Read the model definition and answer for the solid it produces. Units are mm, in the model's axes. A direction names the side the tool comes from. Round coordinates to 2 decimals unless told otherwise and drop trailing zeros. Loops run counter-clockwise (first coordinate to the right, second up) from the corner with the lowest first, then second, coordinate; pieces in that order, holes last. Notation, with made-up numbers: (2, -23.5) - (31, -23.5) arc R31 ccw to (31, 3.5) - close; hole circle Ø4 at (-21, -29). An arc over 180 degrees is marked (long way). Answer as CSV lines item,"result".
```python
from build123d import *

# Parameters (mm, degrees)
F1_DEPTH = 101.6


with BuildPart() as f1:
    # F0 (on Front) → F1 (new body)
    with BuildSketch(Plane.XZ):
        Polygon((-50.8, -32.374417), (50.8, -32.374417), (50.8, 32.374417), (14.084613, 32.374417), (-50.8, 32.374417), align=None)
        with BuildLine():
            Line((14.084613, 32.374417), (50.8, 32.374417))
            Line((50.8, 32.374417), (50.8, 52.120494))
            Line((50.8, 52.120494), (50.8, 74.345494))
            ThreePointArc((50.8, 74.345494), (24.954765, 64.252521), (14.084613, 38.724417))
            Line((14.084613, 38.724417), (14.084613, 32.374417))
        make_face()
        with BuildLine():
            ThreePointArc((50.8, 74.345494), (-5.45833, 66.573015), (-50.8, 32.374417))
            Line((-50.8, 32.374417), (14.084613, 32.374417))
            Line((14.084613, 32.374417), (14.084613, 38.724417))
            ThreePointArc((14.084613, 38.724417), (24.954765, 64.252521), (50.8, 74.345494))
        make_face()
        with BuildLine():
            Line((50.8, 74.345494), (50.8, 52.120494))
            Line((50.8, 52.120494), (90.314029, 52.120494))
            ThreePointArc((90.314029, 52.120494), (94.804157, 53.980366), (96.664029, 58.470494))
            Line((96.664029, 58.470494), (96.664029, 102.920494))
            Line((96.664029, 102.920494), (57.15, 102.920494))
            ThreePointArc((57.15, 102.920494), (52.659872, 101.060622), (50.8, 96.570494))
            Line((50.8, 96.570494), (50.8, 74.345494))
        make_face()
    extrude(amount=F1_DEPTH)


solid = f1.part
```
1) A cutting plane is placed at C-C, the plane x = 69. Determine the outline of the cut face in (y, z).
Entries:
outline,"(-101.6, 52.12) - (0, 52.12) - (0, 102.92) - (-101.6, 102.92) - close"
2) A tool of negligible diameter and unlimited length cuts with its end or side. For faces 1 (the face through (70, -50, 52.12)), 2 (the face through (77, -50, 102.92)), from which of +Z, -Z, +X, -X, +Y, -Y can it reach the whole face along a straight path? Write none if from no direction.
Entries:
face 1,"-Z, +X, +Y, -Y"
face 2,"+Z, +X, -X, +Y, -Y"
3) Find the intervals of material crossed by line 1 (X direction, y = -30.5, z = -22.5); line 2 (X direction, y = -29, z = 88.5); line 3 (Z direction, x = 39.5, y = -61), in increasing order.
Entries:
line 1,"x = -50.8 to 50.8"
line 2,"x = 50.8 to 96.66"
line 3,"z = -32.37 to 75.1"
4) A cutting plane is placed at B-B, the plane z = -13. Determine the outline of the cut face in (x, y), plus the area to 3 significant figures.
Entries:
outline,"(-50.8, -101.6) - (50.8, -101.6) - (50.8, 0) - (-50.8, 0) - close"
area,"10,300 mm^2"
5) A cutting plane is placed at A-A, the plane y = -66. Determine the outline of the cut face in (x, z), plus the area to 3 significant figures.
Entries:
outline,"(-50.8, -32.37) - (50.8, -32.37) - (50.8, 52.12) - (90.31, 52.12) arc R6.35 ccw to (96.66, 58.47) - (96.66, 102.92) - (57.15, 102.92) arc R6.35 ccw to (50.8, 96.57) - (50.8, 74.35) arc R112.81 ccw to (-50.8, 32.37) - close"
area,"12,100 mm^2"
6) Each of these flat-tipped pins is pushed along its axis until it touches: P1, Ø8, axis at x = 14, y = -72, coming from the +Z side; P2, Ø3, axis at y = -66, z = 29.5, coming from the +X side; P3, Ø18, axis at y = -74.5, z = 89, coming from the -X side; P4, Ø1.5, axis at x = 69.5, z = 84.5, coming from the +Y side. Where does it stop, or does it pass through?
Entries:
P1,"stops at z = 73.4"
P2,"stops at x = 50.8"
P3,"stops at x = 50.8"
P4,"stops at y = 0"
